```python
from build123d import *

# Parameters (mm, degrees)
SKETCH2_W          = 33.5
SKETCH2_H          = 40
SKETCH2_R          = 1.5
BASE_FLANGE1_DEPTH = 1.5
FILLET1_R          = 1


# Sheet-metal steps are written as plain solids
with BuildPart() as part:
    # Sketch2 → Base-Flange1 (new body)
    with BuildSketch(Plane.XY):
        with Locations((275.329860694, 200.707229453)):
            Rectangle(SKETCH2_W, SKETCH2_H)
        with Locations((288.579860694, 213.207229453)):
            Circle(SKETCH2_R, mode=Mode.SUBTRACT)
        with Locations((288.579860694, 188.207229453)):
            Circle(SKETCH2_R, mode=Mode.SUBTRACT)
        with Locations((262.079860694, 213.207229453)):
            Circle(SKETCH2_R, mode=Mode.SUBTRACT)
        with Locations((262.079860694, 188.207229453)):
            Circle(SKETCH2_R, mode=Mode.SUBTRACT)
    extrude(amount=-BASE_FLANGE1_DEPTH)

    # Fillet1
    fillet1_edges = [part.edges().sort_by_distance(p)[0] for p in [
        (258.579860694, 220.707229453, -0.75),
        (292.079860694, 220.707229453, -0.75),
        (292.079860694, 180.707229453, -0.75),
        (258.579860694, 180.707229453, -0.75),
    ]]
    fillet(fillet1_edges, radius=FILLET1_R)


solid = part.part
```
Here's how the part is built. I have some questions about the finished solid (model axes, mm). Give positions to 0.01 mm unless a question says otherwise; leave off trailing zeros. Order: outer loops, then holes, each group sorted by start corner. A loop starts at its lowest first (then second) coordinate and runs counter-clockwise, first axis right, second up. Notation, with made-up numbers: M -27.5,37.25 L 7.5,37.25 A16 cw 7.5,66.25 Z; hole C 27.5,19.5 d4. An arc over 180 degrees is marked long. Use a Markdown table: item, result. Add a question column.
1. I need wall thicknesses on probe 1 along Y at (x, z) = (288.5, -1.3); probe 2 along X at (y, z) = (212.5, -0.1); probe 3 along X at (y, z) = (187, -0.45). Which ranges of each line are inside material? Lowest first, please. Write a range as from..to.
2. Suppose I cut it at B-B (x = 262). List the corners of the cut face in (y, z) for me.
3. Suppose I cut it at A-A (z = -1.05). List the corners of the cut face in (x, y) for me, and give its area (3 significant figures).
4. If we mould it in two halves opening along Y, with no side actions, what happens to faces 1 (the cylindrical face through (260.58, 213.27, -0.74)), 2 (the flat face through (292.08, 200, -1)), 3 (the flat face through (275, 220.707, -1))? For each: +Y half, -Y half, draft (parallel to the pull), parting line (faces both ways), or undercut.
Results list:
| question | item | result |
|---|---|---|
| 1 | probe 1 | y = 180.71..186.71, 189.71..211.71, 214.71..220.71 |
| 1 | probe 2 | x = 258.58..260.76, 263.4..287.26, 289.9..292.08 |
| 1 | probe 3 | x = 258.58..261.19, 262.97..287.69, 289.47..292.08 |
| 2 | outline | M 180.71,-1.5 L 186.71,-1.5 L 186.71,0 L 180.71,0 Z; M 189.71,-1.5 L 211.71,-1.5 L 211.71,0 L 189.71,0 Z; M 214.71,-1.5 L 220.71,-1.5 L 220.71,0 L 214.71,0 Z |
| 3 | outline | M 258.58,181.71 A1 ccw 259.58,180.71 L 291.08,180.71 A1 ccw 292.08,181.71 L 292.08,219.71 A1 ccw 291.08,220.71 L 259.58,220.71 A1 ccw 258.58,219.71 Z; hole C 262.08,188.21 d3; hole C 262.08,213.21 d3; hole C 288.58,188.21 d3; hole C 288.58,213.21 d3 |
| 3 | area | 1,310 mm² |
| 4 | face 1 | undercut |
| 4 | face 2 | draft |
| 4 | face 3 | +Y half |
